Source: CAD feature listing. Evaluate the final solid. Frame: model axes, mm. A direction names the side the tool comes from. Give positions to 0.01 mm unless a question says otherwise; leave off trailing zeros. Order: outer loops, then holes, each group sorted by start corner. A loop starts at its lowest first (then second) coordinate and runs counter-clockwise, first axis right, second up. Notation, with made-up numbers: M 6,17.5 L 16,17.5 A12 ccw 16,39.5 Z; hole C 63.5,-4 d8. An arc over 180 degrees is marked long. Answer as a JSON object with one key per item and string values. Group by question number.
1. Section query C-C (y = 9). Output: boundary loops of the cut face in (x, z).
2. Pull-direction query (X, two-part tool) for faces 4 (the flat face through (8, 31, 0)), 5 (the cylindrical face through (0.7, 50.41, 0.91)), 6 (the flat face through (0, 57, 0)); classes: +X half, -X half, draft (parallel to the pull), parting line (faces both ways), or undercut.
3. Section query A-A (z = 0). Output: boundary loops of the cut face in (x, y).
4. Section query D-D (x = 3.5). Output: boundary loops of the cut face in (y, z).
5. Set-up query: faces 1 (the cylindrical face through (12.2, 21.73, -6.34)), 2 (the flat face through (-8, 31, 0)), 3 (the cylindrical face through (0, 1, 5)). Return all of +Z, -Z, +X, -X, +Y, -Y with unobstructed straight access to the full face (end or side cutting, diameter ignored); none if empty.
6. Section query B-B (x = 0). Output: boundary loops of the cut face in (y, z), plus the area to 3 significant figures.
7. Material intervals for L1, parallel to X at y = 34, z = 0; L2, parallel to Y at x = -4, z = 7; L3, parallel to Y at x = 3.5, z = -3.5, sorted ascending. Write a range as [from, to].
8. Pin query (flat end, axial travel): P1, Ø6, axis at x = 3, z = -6, coming from the +Y side; P2, Ø2, axis at x = -8, z = 0, coming from the +Y side; P3, Ø6, axis at y = 15, z = 3.5, coming from the +X side. Return the tip coordinate at first contact, or that it passes through.
from build123d import *

# Parameters (mm, degrees)
SKETCH2_R          = 1.25
CUT_EXTRUDE1_DEPTH = 10


with BuildPart() as part:
    # Sketch1 → Revolve1 (revolve)
    with BuildSketch(Plane(origin=(0, 0, 0), x_dir=(0, 0, -1), z_dir=(1, 0, 0)), mode=Mode.PRIVATE) as revolve1_sk:
        Polygon((0, 57), (-1.15, 57), (-1.15, 44), (-5, 44), (-5, 41), (-13.75, 41), (-13.75, 3), (-5, 3), (-5, 0), (0, 0), align=None)
    revolve(revolve1_sk.sketch.rotate(Axis((0, 0, 0), (0, 1, 0)), 180), axis=Axis((0, 0, 0), (0, 1, 0)))

    # Sketch2 → Cut-Extrude1 (cut)
    with BuildSketch(Plane(origin=(0, 41, 0), x_dir=(1, 0, 0), z_dir=(0, 1, 0))):
        with Locations(Location((-8, 0, 0), (0, 0, 270))):
            Circle(SKETCH2_R)
        with Locations(Location((8, 0, 0), (0, 0, 270))):
            Circle(SKETCH2_R)
    extrude(amount=-CUT_EXTRUDE1_DEPTH, mode=Mode.SUBTRACT)


solid = part.part
Answer sheet:
{
 "1": {"outline": "C 0,0 d27.5"},
 "2": {"face 4": "undercut", "face 5": "parting line", "face 6": "draft"},
 "3": {"outline": "M -13.75,3 L -5,3 L -5,0 L 5,0 L 5,3 L 13.75,3 L 13.75,41 L 9.25,41 L 9.25,31 L 6.75,31 L 6.75,41 L 5,41 L 5,44 L 1.15,44 L 1.15,57 L -1.15,57 L -1.15,44 L -5,44 L -5,41 L -6.75,41 L -6.75,31 L -9.25,31 L -9.25,41 L -13.75,41 Z"},
 "4": {"outline": "M 0,-3.57 L 3,-3.57 L 3,-13.3 L 41,-13.3 L 41,-3.57 L 44,-3.57 L 44,3.57 L 41,3.57 L 41,13.3 L 3,13.3 L 3,3.57 L 0,3.57 Z"},
 "5": {"face 1": "+Y, -Y", "face 2": "+Y", "face 3": "-Y"},
 "6": {"outline": "M 0,-5 L 3,-5 L 3,-13.75 L 41,-13.75 L 41,-5 L 44,-5 L 44,-1.15 L 57,-1.15 L 57,1.15 L 44,1.15 L 44,5 L 41,5 L 41,13.75 L 3,13.75 L 3,5 L 0,5 Z", "area": "1,130 mm^2"},
 "7": {"L1": "[-13.75, -9.25], [-6.75, 6.75], [9.25, 13.75]", "L2": "[3, 41]", "L3": "[0, 44]"},
 "8": {"P1": "y = 44", "P2": "y = 31", "P3": "x = 13.74"}
}
